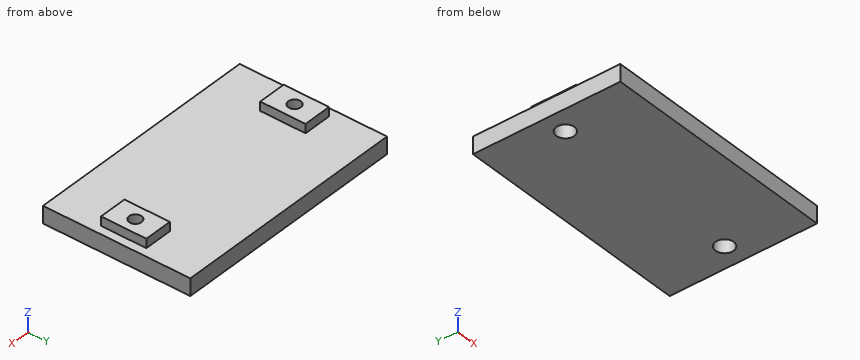
```python
from build123d import *

# Parameters (mm, degrees)
MOUNTING_PLATE_SKETCH_W       = 42
MOUNTING_PLATE_SKETCH_H       = 26
MOUNTING_PLATE_DEPTH          = 3
CLAMP_SEAT_1_SKETCH_W         = 5
CLAMP_SEAT_1_SKETCH_H         = 8
CLAMP_SEAT_1_DEPTH            = 1.7
M2_SCREW_CLEARANCE_1_SKETCH_R = 1.1
M2_SCREW_CLEARANCE_1_DEPTH    = 4.8
M2_INSERT_POCKET_1_SKETCH_R   = 1.6
M2_INSERT_POCKET_1_DEPTH      = 2.5
CLAMP_SEAT_2_SKETCH_W         = 5
CLAMP_SEAT_2_SKETCH_H         = 8
CLAMP_SEAT_2_DEPTH            = 1.7
M2_SCREW_CLEARANCE_2_SKETCH_R = 1.1
M2_SCREW_CLEARANCE_2_DEPTH    = 4.8
M2_INSERT_POCKET_2_SKETCH_R   = 1.6
M2_INSERT_POCKET_2_DEPTH      = 2.5


with BuildPart() as part:
    # Mounting Plate Sketch → Mounting Plate (new body)
    with BuildSketch(Plane.XY):
        Rectangle(MOUNTING_PLATE_SKETCH_W, MOUNTING_PLATE_SKETCH_H)
    extrude(amount=MOUNTING_PLATE_DEPTH)

    # Clamp Seat 1 Sketch → Clamp Seat 1 (add)
    with BuildSketch(Plane.XY.offset(2.9)):
        with Locations((-17, 0)):
            Rectangle(CLAMP_SEAT_1_SKETCH_W, CLAMP_SEAT_1_SKETCH_H)
    extrude(amount=CLAMP_SEAT_1_DEPTH)

    # M2 Screw Clearance 1 Sketch → M2 Screw Clearance 1 (cut)
    with BuildSketch(Plane.XY.offset(-0.1)):
        with Locations((-17, 0)):
            Circle(M2_SCREW_CLEARANCE_1_SKETCH_R)
    extrude(amount=M2_SCREW_CLEARANCE_1_DEPTH, mode=Mode.SUBTRACT)

    # M2 Insert Pocket 1 Sketch → M2 Insert Pocket 1 (cut)
    with BuildSketch(Plane.XY.offset(-0.1)):
        with Locations((-17, 0)):
            Circle(M2_INSERT_POCKET_1_SKETCH_R)
    extrude(amount=M2_INSERT_POCKET_1_DEPTH, mode=Mode.SUBTRACT)

    # Clamp Seat 2 Sketch → Clamp Seat 2 (add)
    with BuildSketch(Plane.XY.offset(2.9)):
        with Locations((17, 0)):
            Rectangle(CLAMP_SEAT_2_SKETCH_W, CLAMP_SEAT_2_SKETCH_H)
    extrude(amount=CLAMP_SEAT_2_DEPTH)

    # M2 Screw Clearance 2 Sketch → M2 Screw Clearance 2 (cut)
    with BuildSketch(Plane.XY.offset(-0.1)):
        with Locations((17, 0)):
            Circle(M2_SCREW_CLEARANCE_2_SKETCH_R)
    extrude(amount=M2_SCREW_CLEARANCE_2_DEPTH, mode=Mode.SUBTRACT)

    # M2 Insert Pocket 2 Sketch → M2 Insert Pocket 2 (cut)
    with BuildSketch(Plane.XY.offset(-0.1)):
        with Locations((17, 0)):
            Circle(M2_INSERT_POCKET_2_SKETCH_R)
    extrude(amount=M2_INSERT_POCKET_2_DEPTH, mode=Mode.SUBTRACT)


solid = part.part
```
Can you work these out from the model? Positions are in its coordinate system, mm. Coordinates: 2 decimals unless noted, no trailing zeros. Loops run counter-clockwise (first coordinate to the right, second up) from the corner with the lowest first, then second, coordinate; pieces in that order, holes last.
1) Imagine slicing it at A-A on y = 0. List the corners of the cut face in (x, z) for me.
2) Imagine slicing it at B-B on z = 3.65. List the corners of the cut face in (x, y) for me, plus the area to 3 significant figures.
3) Imagine slicing it at C-C on x = 17. List the corners of the cut face in (y, z) for me.
4) Imagine slicing it at D-D on y = -2.75. List the corners of the cut face in (x, z) for me, plus the area to 3 significant figures.
5) For pin 1 (0.8 mm diameter, centred on y = 0.5, z = 4, fed in from +X); pin 2 (3 mm diameter, centred on x = -5, y = 1, fed in from +Z); pin 3 (1.8 mm diameter, centred on x = 16.5, z = 4, fed in from -Y), each with a flat end and sliding along its axis, tell me the tip position at first contact or that it passes through.
6) I need wall thicknesses on probe 1 along X at (y, z) = (0, 4.15); probe 2 along X at (y, z) = (0, 1.4); probe 3 along Y at (x, z) = (-17, 3.35). Which ranges of each line are inside material? Lowest first, please.
Completed:
1. outline: (-21, 0) - (-18.6, 0) - (-18.6, 2.4) - (-18.1, 2.4) - (-18.1, 4.6) - (-19.5, 4.6) - (-19.5, 3) - (-21, 3) - close; (-15.9, 2.4) - (-15.4, 2.4) - (-15.4, 0) - (15.4, 0) - (15.4, 2.4) - (15.9, 2.4) - (15.9, 4.6) - (14.5, 4.6) - (14.5, 3) - (-14.5, 3) - (-14.5, 4.6) - (-15.9, 4.6) - close; (18.1, 2.4) - (18.6, 2.4) - (18.6, 0) - (21, 0) - (21, 3) - (19.5, 3) - (19.5, 4.6) - (18.1, 4.6) - close
2. outline: (-19.5, -4) - (-14.5, -4) - (-14.5, 4) - (-19.5, 4) - close; (14.5, -4) - (19.5, -4) - (19.5, 4) - (14.5, 4) - close; hole circle Ø2.2 at (-17, 0); hole circle Ø2.2 at (17, 0)
2. area: 72.4 mm2
3. outline: (-13, 0) - (-1.6, 0) - (-1.6, 2.4) - (-1.1, 2.4) - (-1.1, 4.6) - (-4, 4.6) - (-4, 3) - (-13, 3) - close; (1.1, 2.4) - (1.6, 2.4) - (1.6, 0) - (13, 0) - (13, 3) - (4, 3) - (4, 4.6) - (1.1, 4.6) - close
4. outline: (-21, 0) - (21, 0) - (21, 3) - (19.5, 3) - (19.5, 4.6) - (14.5, 4.6) - (14.5, 3) - (-14.5, 3) - (-14.5, 4.6) - (-19.5, 4.6) - (-19.5, 3) - (-21, 3) - close
4. area: 142 mm2
5. pin 1: stops at x = 19.5
5. pin 2: stops at z = 3
5. pin 3: stops at y = -4
6. probe 1: x = -19.5 to -18.1, -15.9 to -14.5, 14.5 to 15.9, 18.1 to 19.5
6. probe 2: x = -21 to -18.6, -15.4 to 15.4, 18.6 to 21
6. probe 3: y = -4 to -1.1, 1.1 to 4
